Verification items for the finished model (mm, model axes). Face numbers are marked on the shaded views. A direction names the side the tool comes from. Give positions to 0.01 mm unless a question says otherwise; leave off trailing zeros. Write each loop counter-clockwise with the first axis right and the second up, starting at its lowest first coordinate (ties: lowest second). Pieces come first, ordered by that corner, then holes. Notation, with made-up numbers: M 10.5,-38.75 L 17.5,-38.75 A19 ccw 17.5,-33.75 Z; hole C 71.5,3 d1. An arc over 180 degrees is marked long. Answer as a JSON object with one key per item and string values.
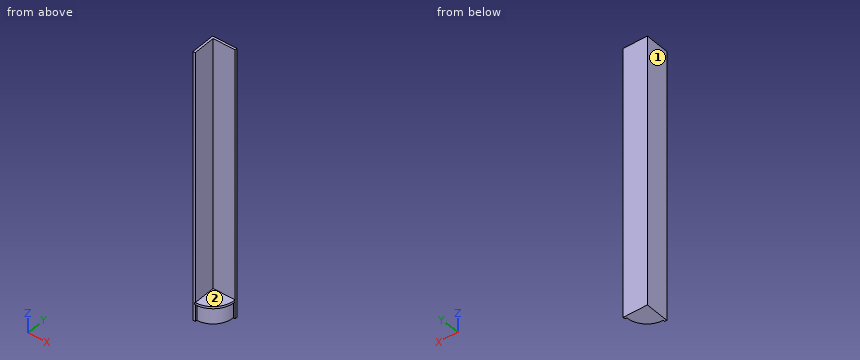
```python
from build123d import *

# Parameters (mm, degrees)
F1_DEPTH = 2110
F3_DEPTH = 18
F5_DEPTH = 140


with BuildPart() as f1:
    # F0 (on Top) → F1 (new body)
    with BuildSketch(Plane.XY):
        Polygon((-318.834358, 154.102758), (-518.834358, 154.102758), (-518.834358, -45.897242), (-500.834358, -45.897242), (-500.834358, 136.102758), (-336.834358, 136.102758), (-318.834358, 136.102758), align=None)
    extrude(amount=F1_DEPTH)

    # F2 (on Top) → F3 (join)
    with BuildSketch(Plane.XY):
        with BuildLine():
            Line((-318.834358, 154.102758), (-518.834358, 154.102758))
            Line((-518.834358, 154.102758), (-518.834358, -45.897242))
            Line((-518.834358, -45.897242), (-506.854117, -45.897242))
            ThreePointArc((-506.854117, -45.897242), (-374.280698, 5.263707), (-318.834358, 136.102758))
            Line((-318.834358, 136.102758), (-318.834358, 154.102758))
        make_face()
    extrude(amount=F3_DEPTH)

    # F4 (on Top) → F5 (join)
    with BuildSketch(Plane.XY):
        with BuildLine():
            Line((-318.834358, 154.102758), (-518.834358, 154.102758))
            Line((-518.834358, 154.102758), (-518.834358, -45.897242))
            Line((-518.834358, -45.897242), (-500.834358, -45.897242))
            Line((-500.834358, -45.897242), (-500.834358, -30.897242))
            ThreePointArc((-500.834358, -30.897242), (-382.747526, 18.015926), (-333.834358, 136.102758))
            Line((-333.834358, 136.102758), (-318.834358, 136.102758))
            Line((-318.834358, 136.102758), (-318.834358, 154.102758))
        make_face()
    extrude(amount=-F5_DEPTH)


solid = f1.part
```
1) Go/stop test with flat-tipped pins: pin 1 (12 mm diameter, centred on x = -401, y = 45.5, fed in from +Z); pin 2 (4.5 mm diameter, centred on x = -325, z = -39.5, fed in from -Y); pin 3 (12 mm diameter, centred on y = 53.5, z = 385, fed in from +X). Record where each tip stops, or that it passes through.
Completed:
{"pin 1": "stops at z = 18", "pin 2": "stops at y = 136.1", "pin 3": "stops at x = -500.83"}
2) Thickness scan on L1, parallel to X at y = 19.5, z = 284; L2, parallel to Z at x = -474.5, y = 102.5; L3, parallel to Y at x = -404.5, z = 159. Record the ranges inside material, lowest first.
Completed:
{"L1": "x = -518.83 to -500.83", "L2": "z = -140 to 18", "L3": "y = 136.1 to 154.1"}
3) Access from +Z, -Z, +X, -X, +Y, -Y to the whole of each face (thin tool, end or side, straight path). Record for the marked faces 1 and 2.
Completed:
{"face 1": "+Z, -Z, -X, +Y, -Y", "face 2": "+Z, +X, -Y"}
4) Section check B-B on x = -396. Record the boundary of the cut face in (y, z).
Completed:
{"outline": "M -12.72,0 L 6.11,0 L 6.11,-140 L 154.1,-140 L 154.1,2110 L 136.1,2110 L 136.1,18 L -12.72,18 Z"}
5) Section check A-A on z = 1058. Record the boundary of the cut face in (x, y), and give its area (3 significant figures).
Completed:
{"outline": "M -518.83,-45.9 L -500.83,-45.9 L -500.83,136.1 L -318.83,136.1 L -318.83,154.1 L -518.83,154.1 Z", "area": "6,880 mm2"}
6) Section check C-C on y = 75. Record the boundary of the cut face in (x, z).
Completed:
{"outline": "M -518.83,-140 L -345.41,-140 L -345.41,0 L -329.39,0 L -329.39,18 L -500.83,18 L -500.83,2110 L -518.83,2110 Z"}
